Part print with two shaded views. Sizes in mm from the minimum x, y, z corner. A direction names the side the tool comes from. Round coordinates to 2 decimals unless told otherwise and drop trailing zeros. Write each loop counter-clockwise with the first axis right and the second up, starting at its lowest first coordinate (ties: lowest second). Pieces come first, ordered by that corner, then holes. Notation, with made-up numbers: (51, 34.25) -> (95, 34.25) arc R25 cw to (95, 59.25) -> close; hole circle Ø3 at (-33, 25). An arc over 180 degrees is marked (long way). Answer as CSV lines item,"result".
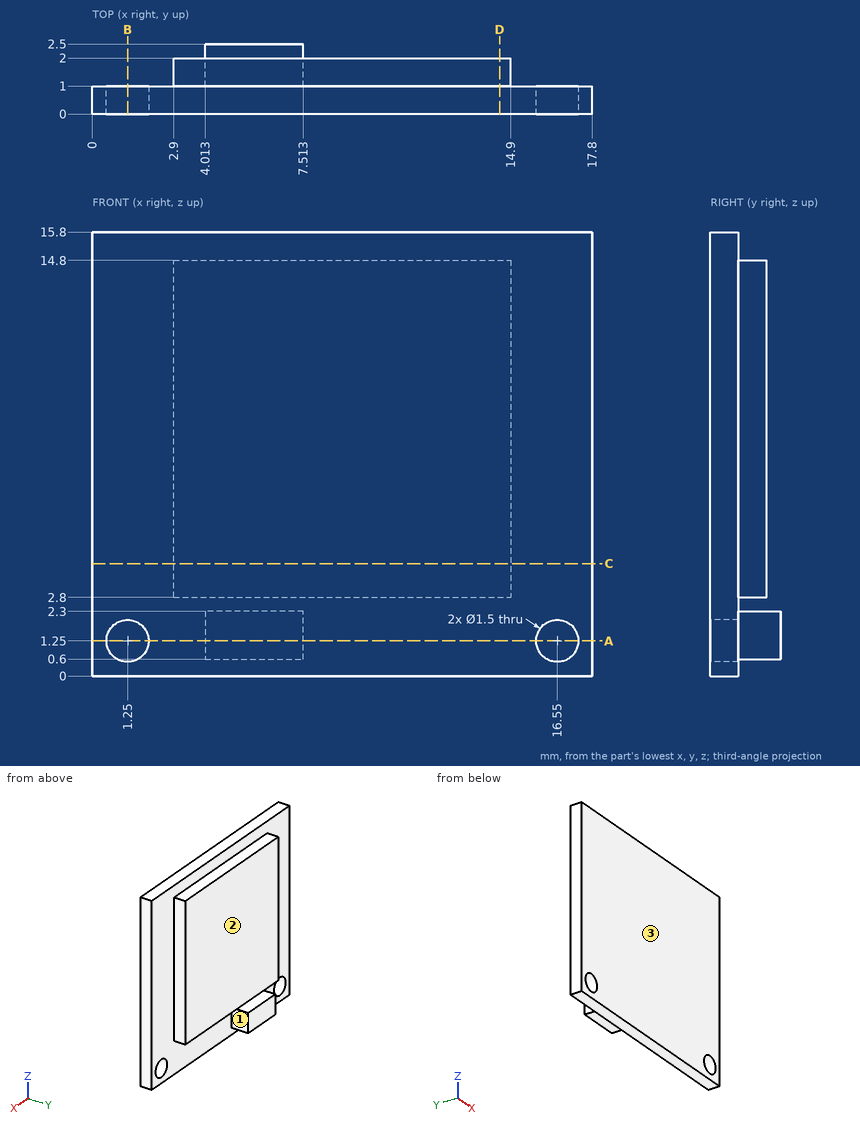
1. Cut at A-A, the plane z = 1.25. Write the cut outline in (x, y).
Results found:
outline,"(0, 0) -> (0.5, 0) -> (0.5, 1) -> (0, 1) -> close; (2, 0) -> (15.8, 0) -> (15.8, 1) -> (7.51, 1) -> (7.51, 2.5) -> (4.01, 2.5) -> (4.01, 1) -> (2, 1) -> close; (17.3, 0) -> (17.8, 0) -> (17.8, 1) -> (17.3, 1) -> close"
2. Cut at D-D, the plane x = 14.5. Write the cut outline in (y, z), then the cut area to 3 significant figures.
Results found:
outline,"(0, 0) -> (1, 0) -> (1, 2.8) -> (2, 2.8) -> (2, 14.8) -> (1, 14.8) -> (1, 15.8) -> (0, 15.8) -> close"
area,"27.8 mm2"
3. Drop flat-ended pins along their axis: pin 1 Ø1.7 at (x, z) = (1.25, 1.25) entering from +Y; pin 2 Ø5 at (x, z) = (4.5, 2) entering from -Y; pin 3 Ø0.5 at (y, z) = (1.5, 9.5) entering from +X; pin 4 Ø0.8 at (x, y) = (10, 1.5) entering from -Z. Give the stop position or say it passes through.
Results found:
pin 1,"stops at y = 1"
pin 2,"stops at y = 0"
pin 3,"stops at x = 14.9"
pin 4,"stops at z = 2.8"
4. Probe line 1 along Z through (x, y) = (1.25, 0.5); line 2 along Y through (x, z) = (4.75, 8.5); line 3 along Y through (x, z) = (14, 1). List the from-to ranges inside material, lowest first.
Results found:
line 1,"z = 0 to 0.5, 2 to 15.8"
line 2,"y = 0 to 2"
line 3,"y = 0 to 1"
5. Cut at B-B, the plane x = 1.25. Write the cut outline in (y, z), then the cut area to 3 significant figures.
Results found:
outline,"(0, 0) -> (1, 0) -> (1, 0.5) -> (0, 0.5) -> close; (0, 2) -> (1, 2) -> (1, 15.8) -> (0, 15.8) -> close"
area,"14.3 mm2"
6. Cut at C-C, the plane z = 4. Write the cut outline in (x, y).
Results found:
outline,"(0, 0) -> (17.8, 0) -> (17.8, 1) -> (14.9, 1) -> (14.9, 2) -> (2.9, 2) -> (2.9, 1) -> (0, 1) -> close"
7. Which spindle directions (+Z, -Z, +X, -X, +Y, -Y) get a long thin tool onto all of the face, cutting with end or side? Do the marked faces 1, 2 and 3. Say none if no direction does.
Results found:
face 1,"-Z, +X, +Y"
face 2,"+Z, +X, -X, +Y"
face 3,"+Z, -Z, +X, -X, -Y"
